Input: dimensioned drawing with shaded views. Units: mm. Origin: part minimum x, y, z. A direction names the side the tool comes from. Give positions to 0.01 mm unless a question says otherwise; leave off trailing zeros. Write each loop counter-clockwise with the first axis right and the second up, starting at its lowest first coordinate (ties: lowest second). Pieces come first, ordered by that corner, then holes. Notation, with made-up numbers: (-12, -4.75) -> (2, -4.75) arc R31 ccw to (2, 32.25) -> close; hole circle Ø6 at (-28, 37.25). An arc over 180 degrees is marked (long way). Return JSON: item names as keys, results as strings. Group by question number.
Item 1: Section A-A, the plane y = 36. Return loops of the section in (x, z), then the cut area to 3 significant figures.
Item 2: Section B-B, the plane x = 10. Return loops of the section in (y, z).
Item 3: Pin query (flat end, axial travel): P1, Ø3, axis at x = 9, y = 12, coming from the -Z side; P2, Ø10, axis at x = 14.5, z = 17, coming from the +Y side; P3, Ø2, axis at x = 4, z = 16.5, coming from the -Y side; P4, Ø7.5, axis at x = 10, y = 36, coming from the +Z side. Return the tip coordinate at first contact, or that it passes through.
Item 4: Line query: line 1 (Y direction, x = 10, z = 28.55); line 2 (Y direction, x = 19.25, z = 10.5); line 3 (Z direction, x = 8.25, y = 18.5). Output: solid intervals per line, ascending. Write a range as [from, to].
Item 5: Section D-D, the plane y = 10.5. Return loops of the section in (x, z).
Item 6: Section C-C, the plane x = 16.75. Return loops of the section in (y, z), then the cut area to 3 significant figures.
Item 7: Mould query, pull axis X, two halves, no side actions, for the marked faces 4, 5 and 6. Classes: released by +X, released by -X, zero draft, split by the parting line, or undercut.
Item 8: Set-up query: the marked faces 1, 2 and 3. Return all of +Z, -Z, +X, -X, +Y, -Y with unobstructed straight access to the full face (end or side cutting, diameter ignored); none if empty.
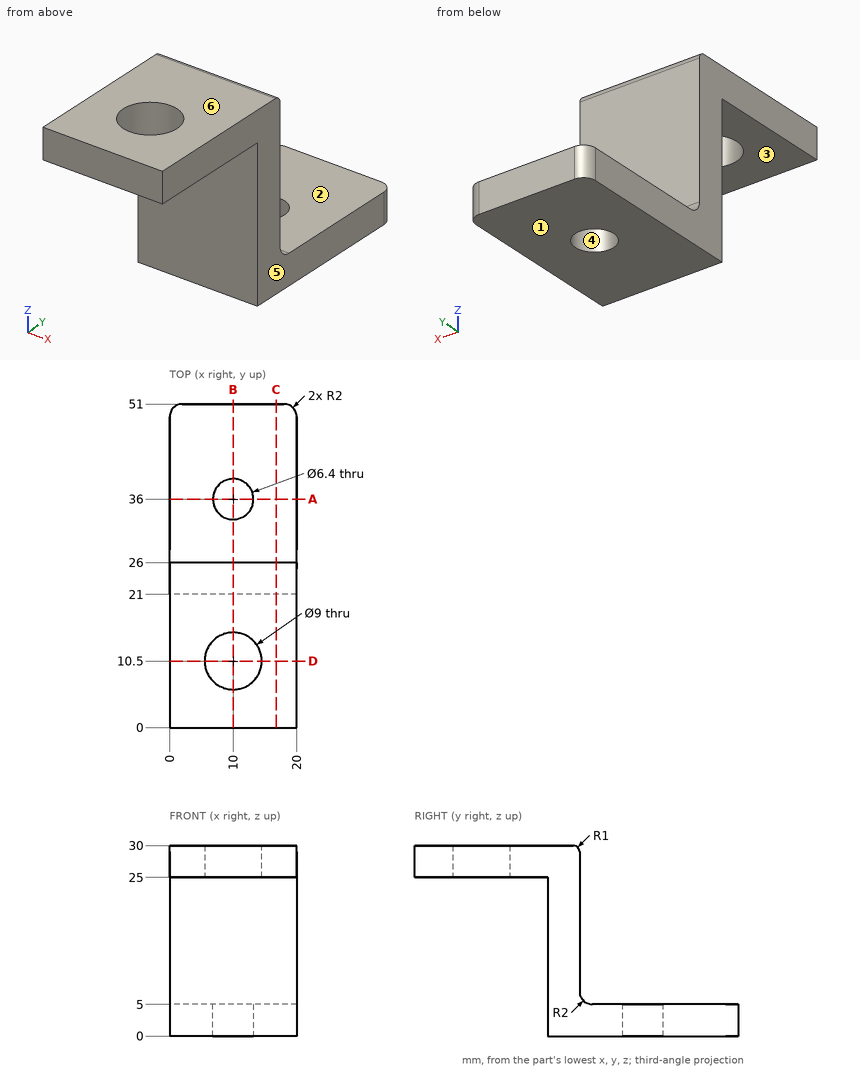
Answer below:
{
 "1": {"outline": "(0, 0) -> (6.8, 0) -> (6.8, 5) -> (0, 5) -> close; (13.2, 0) -> (20, 0) -> (20, 5) -> (13.2, 5) -> close", "area": "68.0 mm2"},
 "2": {"outline": "(0, 25) -> (6, 25) -> (6, 30) -> (0, 30) -> close; (15, 25) -> (21, 25) -> (21, 0) -> (32.8, 0) -> (32.8, 5) -> (28, 5) arc R2 cw to (26, 7) -> (26, 29) arc R1 ccw to (25, 30) -> (15, 30) -> close; (39.2, 0) -> (51, 0) -> (51, 5) -> (39.2, 5) -> close"},
 "3": {"P1": "passes through", "P2": "stops at y = 26", "P3": "stops at y = 21", "P4": "stops at z = 5"},
 "4": {"line 1": "y = [0, 6], [15, 26]", "line 2": "y = [21, 26]", "line 3": "z = [25, 30]"},
 "5": {"outline": "(0, 25) -> (5.5, 25) -> (5.5, 30) -> (0, 30) -> close; (14.5, 25) -> (20, 25) -> (20, 30) -> (14.5, 30) -> close"},
 "6": {"outline": "(0, 25) -> (21, 25) -> (21, 0) -> (51, 0) -> (51, 5) -> (28, 5) arc R2 cw to (26, 7) -> (26, 29) arc R1 ccw to (25, 30) -> (0, 30) -> close", "area": "381 mm2"},
 "7": {"face 4": "undercut", "face 5": "released by +X", "face 6": "zero draft"},
 "8": {"face 1": "-Z, +X, -X, +Y, -Y", "face 2": "+Z, +X, -X, +Y", "face 3": "-Z, +X, -X, -Y"}
}
